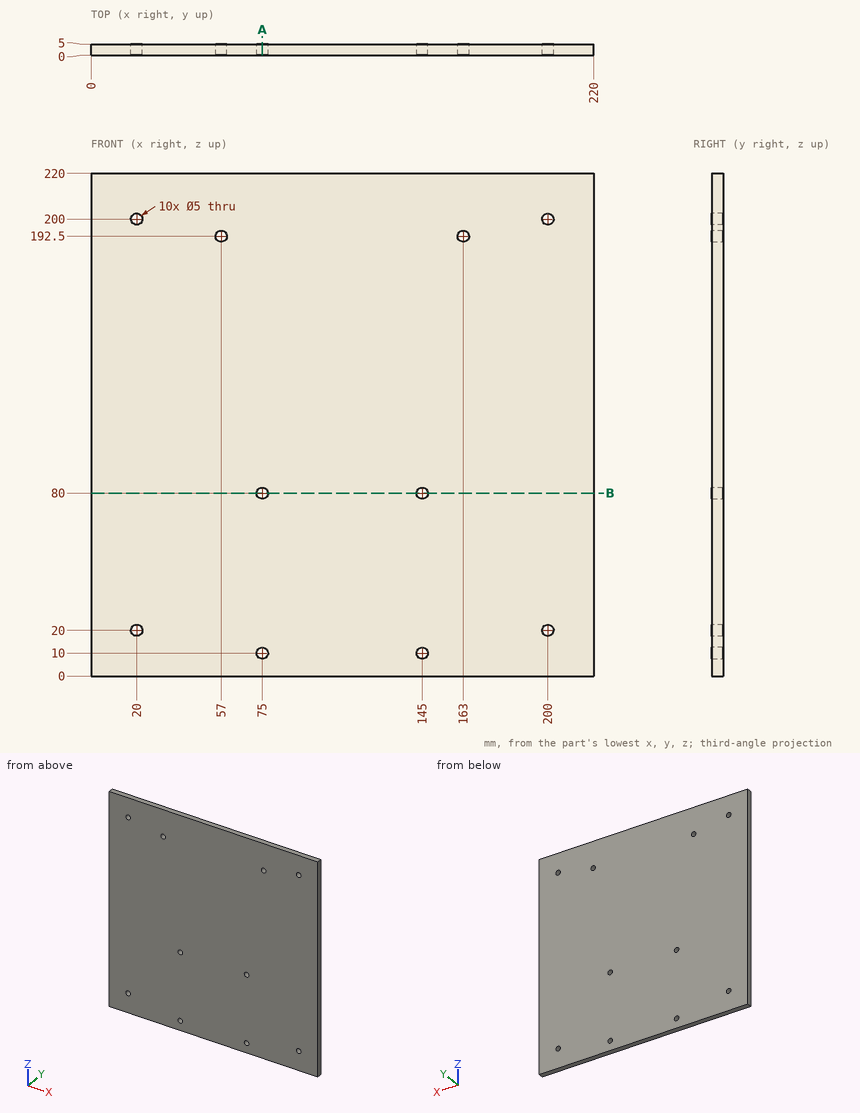
The figure shows three views and two pictorial views of one solid part (mm, origin at its lowest corner). Answer the questions. Coordinates: 2 decimals unless noted, no trailing zeros. Loops run counter-clockwise (first coordinate to the right, second up) from the corner with the lowest first, then second, coordinate; pieces in that order, holes last.
1) Find section B-B on z = 80. Write down the section's boundary in (x, y).
2) Find the intervals of material crossed by L1, parallel to X at y = 2.95, z = 20; L2, parallel to Z at x = 145, y = 3.2; L3, parallel to X at y = 1.25, z = 192.5, in increasing order.
3) Find section A-A on x = 75. Write down the section's boundary in (y, z).
Values:
1. outline: (0, 0) - (72.5, 0) - (72.5, 5) - (0, 5) - close; (77.5, 0) - (142.5, 0) - (142.5, 5) - (77.5, 5) - close; (147.5, 0) - (220, 0) - (220, 5) - (147.5, 5) - close
2. L1: x = 0 to 17.5, 22.5 to 197.5, 202.5 to 220
2. L2: z = 0 to 7.5, 12.5 to 77.5, 82.5 to 220
2. L3: x = 0 to 54.5, 59.5 to 160.5, 165.5 to 220
3. outline: (0, 0) - (5, 0) - (5, 7.5) - (0, 7.5) - close; (0, 12.5) - (5, 12.5) - (5, 77.5) - (0, 77.5) - close; (0, 82.5) - (5, 82.5) - (5, 220) - (0, 220) - close
